Work out the finished part from the listing and answer in its coordinate system (mm). A direction names the side the tool comes from. Coordinates: 2 decimals unless noted, no trailing zeros. Loops run counter-clockwise (first coordinate to the right, second up) from the corner with the lowest first, then second, coordinate; pieces in that order, holes last. Notation, with made-up numbers: (73.5, 75) - (90.5, 75) arc R34 cw to (90.5, 111) - close; hole circle Ø9 at (-6, 20.25). An arc over 180 degrees is marked (long way). Write each question's results on one line, items separated by ' | '. Start each with the question number.
Item 1: Each of these flat-tipped pins is pushed along its axis until it touches: pin 1 Ø2 at (x, z) = (3.5, 24) entering from +Y; pin 2 Ø8 at (x, y) = (7.5, 14) entering from +Z; pin 3 Ø10 at (x, z) = (4, 15.5) entering from +Y. Where does it stop, or does it pass through?
Item 2: For a pull along Y with two mould halves and no side action, classify faces 1 (the face through (-4.14, 33.406, 25.493)), 2 (the face through (1, 9, 23)), 3 (the face through (1, 18, 17)) as +Y half, -Y half, draft (parallel to the pull), parting line (faces both ways), or undercut.
Item 3: Section D-D, the plane z = 19.5 is taken. Write down the section's boundary in (x, y).
Item 4: A tool of negligible diameter and unlimited length cuts with its end or side. For faces 4 (the face through (4.571, -5.819, 23.225)), 5 (the face through (-0.5, 16.8, 14.5)), from which of +Z, -Z, +X, -X, +Y, -Y can it reach the whole face along a straight path? Write none if from no direction.
Item 5: Section C-C, the plane z = 15.5 is taken. Write down the section's boundary in (x, y), plus the area to 3 significant figures.
Item 6: Section B-B, the plane x = 1.28 is taken. Write down the section's boundary in (y, z), plus the area to 3 significant figures.
Item 7: Consider probe 1 along Z at (x, y) = (-2, 14); probe 2 along Z at (x, y) = (7, 28); probe 3 along Y at (x, z) = (3, 24.25). Determine where each line is inside the solid, lowest interval first. Write a range as [from, to].
Item 8: Section A-A, the plane y = 9 is taken. Write down the section's boundary in (x, z).
from build123d import *

# Parameters (mm, degrees)
FILLET017_R               = 1
FILLET018_R               = 1
FILLET019_R               = 2
FILLET020_R               = 1
FILLET020_PLACEMENT_ANGLE = 180


with BuildPart() as cone010:
    # Cone010 → Cone010 (revolve)
    with BuildSketch(Plane.XZ):
        Polygon((0, 0), (19, 0), (15, 5), (0, 5), align=None)
    revolve(axis=Axis((0, 0, 0), (0, 0, 1)))


with BuildPart() as fillet020:
    # Sketch013 → Revolve (revolve)
    with BuildSketch(Plane.XZ):
        Polygon((0, 0), (-25, 0), (-25, 4), (-23, 4), (-21, 11), (-8, 11), (-8, 17), (0, 17), align=None)
    revolve(axis=Axis((0, 0, 0), (0, 0, 1)))

    # Fillet017
    fillet017_edges = [fillet020.edges().sort_by_distance(p)[0] for p in [
        (21, 0, 11),
        (8, 0, 17),
    ]]
    fillet(fillet017_edges, radius=FILLET017_R)

    # Fillet018
    fillet018_edges = [fillet020.edges().sort_by_distance(p)[0] for p in [
        (25, 0, 4),
    ]]
    fillet(fillet018_edges, radius=FILLET018_R)

    # Fillet019
    fillet019_edges = [fillet020.edges().sort_by_distance(p)[0] for p in [
        (25, 0, 0),
    ]]
    fillet(fillet019_edges, radius=FILLET019_R)

    # Cut014: cut Cone010
    add(cone010.part, mode=Mode.SUBTRACT)

    # Fillet020
    fillet020_edges = [fillet020.edges().sort_by_distance(p)[0] for p in [
        (-19, 0, 0),
    ]]
    fillet(fillet020_edges, radius=FILLET020_R)


with BuildPart() as fillet020_1:
    # Fillet020 placement: moved
    add(fillet020.part.moved(Location((1.28, 9, 28))).rotate(Axis((1.28, 9, 28), (0, 1, 0)), FILLET020_PLACEMENT_ANGLE))


solid = fillet020_1.part
Answer key:
1) pin 1: stops at y = 33.93 | pin 2: stops at z = 23 | pin 3: stops at y = 30.91
2) face 1: parting line | face 2: undercut | face 3: draft
3) outline: circle Ø43.43 at (1.28, 9)
4) face 4: +Z | face 5: -Z
5) outline: circle Ø16 at (1.28, 9) | area: 201 mm^2
6) outline: (-16, 25) arc R1 ccw to (-15, 24) - (-14, 24) - (-12.21, 17.73) arc R1 ccw to (-11.25, 17) - (1, 17) - (1, 12) arc R1 ccw to (2, 11) - (16, 11) arc R1 ccw to (17, 12) - (17, 17) - (29.25, 17) arc R1 ccw to (30.21, 17.73) - (32, 24) - (33, 24) arc R1 ccw to (34, 25) - (34, 26) arc R2 ccw to (32, 28) - (28.48, 28) arc R1 ccw to (27.7, 27.62) - (24, 23) - (-6, 23) - (-9.7, 27.62) arc R1 ccw to (-10.48, 28) - (-14, 28) arc R2 ccw to (-16, 26) - close | area: 431 mm^2
7) probe 1: z = [11, 23] | probe 2: z = [17, 28] | probe 3: y = [-15.6, -6.91], [24.91, 33.6]
8) outline: (-23.72, 25) arc R1 ccw to (-22.72, 24) - (-21.72, 24) - (-19.93, 17.73) arc R1 ccw to (-18.97, 17) - (-6.72, 17) - (-6.72, 12) arc R1 ccw to (-5.72, 11) - (8.28, 11) arc R1 ccw to (9.28, 12) - (9.28, 17) - (21.53, 17) arc R1 ccw to (22.49, 17.73) - (24.28, 24) - (25.28, 24) arc R1 ccw to (26.28, 25) - (26.28, 26) arc R2 ccw to (24.28, 28) - (20.76, 28) arc R1 ccw to (19.98, 27.62) - (16.28, 23) - (-13.72, 23) - (-17.42, 27.62) arc R1 ccw to (-18.2, 28) - (-21.72, 28) arc R2 ccw to (-23.72, 26) - close
